```python
from build123d import *

# Parameters (mm, degrees)
SKETCH1_W           = 82
SKETCH1_H           = 37.5
BOSS_EXTRUDE2_DEPTH = 2
SKETCH2_W           = 3
SKETCH2_H           = 37.5
BOSS_EXTRUDE4_DEPTH = 3
BOSS_EXTRUDE5_DEPTH = 31
SKETCH6_W           = 16.5
SKETCH6_H           = 8
CUT_EXTRUDE1_DEPTH  = 2
SKETCH7_W           = 28.5
SKETCH7_H           = 25
CUT_EXTRUDE2_DEPTH  = 2
SKETCH8_W           = 0.8
SKETCH8_H           = 0.8
BOSS_EXTRUDE6_DEPTH = 5
SKETCH9_W           = 35
SKETCH9_H           = 2
BOSS_EXTRUDE7_DEPTH = 2.4


with BuildPart() as part:
    # Sketch1 → Boss-Extrude2 (new body)
    with BuildSketch(Plane(origin=(0, 0, 0), x_dir=(1, 0, 0), z_dir=(0, 1, 0))):
        with Locations((41, 18.75)):
            Rectangle(SKETCH1_W, SKETCH1_H)
    extrude(amount=BOSS_EXTRUDE2_DEPTH)

    # Sketch2 → Boss-Extrude4 (add)
    with BuildSketch(Plane(origin=(0, 2, 0), x_dir=(1, 0, 0), z_dir=(0, 1, 0))):
        with Locations((9.5, 18.75)):
            Rectangle(SKETCH2_W, SKETCH2_H)
        with Locations((68.5, 18.75)):
            Rectangle(SKETCH2_W, SKETCH2_H)
    extrude(amount=BOSS_EXTRUDE4_DEPTH)

    # Sketch4 → Boss-Extrude5 (add)
    with BuildSketch(Plane(origin=(0, 2, 0), x_dir=(1, 0, 0), z_dir=(0, 1, 0))):
        Polygon((11, 37.5), (8, 37.5), (0, 37.5), (0, 0), (8, 0), (11, 0), (67, 0), (70, 0), (82, 0), (82, 37.5), (70, 37.5), (67, 37.5), align=None)
        Polygon((2, 2), (2, 35.5), (8, 35.5), (11, 35.5), (67, 35.5), (70, 35.5), (80, 35.5), (80, 2), (70, 2), (67, 2), (11, 2), (8, 2), align=None, mode=Mode.SUBTRACT)
    extrude(amount=BOSS_EXTRUDE5_DEPTH)

    # Sketch6 → Cut-Extrude1 (cut)
    with BuildSketch(Plane.ZY):
        with Locations((-18.75, 29)):
            Rectangle(SKETCH6_W, SKETCH6_H)
    extrude(amount=-CUT_EXTRUDE1_DEPTH, mode=Mode.SUBTRACT)

    # Sketch7 → Cut-Extrude2 (cut)
    with BuildSketch(Plane(origin=(82, 0, 0), x_dir=(0, 0, -1), z_dir=(1, 0, 0))):
        with Locations((18.75, 17.5)):
            Rectangle(SKETCH7_W, SKETCH7_H)
    extrude(amount=-CUT_EXTRUDE2_DEPTH, mode=Mode.SUBTRACT)

    # Sketch8 → Boss-Extrude6 (add)
    with BuildSketch(Plane(origin=(2, 0, 0), x_dir=(0, 0, -1), z_dir=(1, 0, 0))):
        with Locations((7.65, 28.2)):
            Rectangle(SKETCH8_W, SKETCH8_H)
        with Locations((29.85, 28.2)):
            Rectangle(SKETCH8_W, SKETCH8_H)
    extrude(amount=BOSS_EXTRUDE6_DEPTH)

    # Sketch9 → Boss-Extrude7 (add)
    with BuildSketch(Plane(origin=(0, 0, -37.5), x_dir=(-1, 0, 0), z_dir=(0, 0, -1))):
        with Locations((-55.5, 26)):
            Rectangle(SKETCH9_W, SKETCH9_H)
        with Locations((-55.5, 5)):
            Rectangle(SKETCH9_W, SKETCH9_H)
    extrude(amount=BOSS_EXTRUDE7_DEPTH)


solid = part.part
```
Input: part model. Units: mm. Frame: model coordinates. A direction names the side the tool comes from. Give positions to 0.01 mm unless a question says otherwise; leave off trailing zeros. Order: outer loops, then holes, each group sorted by start corner. A loop starts at its lowest first (then second) coordinate and runs counter-clockwise, first axis right, second up. Notation, with made-up numbers: (39, -36.5) - (43, -36.5) arc R18 cw to (43, -28.5) - close; hole circle Ø10 at (48, -37.75). An arc over 180 degrees is marked (long way). Use a Markdown table: item, result.
(1) Section query B-B (x = 40). Output: boundary loops of the cut face in (y, z), then the cut area to 3 significant figures.
Computed values:
| item | result |
|---|---|
| outline | (0, -37.5) - (4, -37.5) - (4, -39.9) - (6, -39.9) - (6, -37.5) - (25, -37.5) - (25, -39.9) - (27, -39.9) - (27, -37.5) - (33, -37.5) - (33, -35.5) - (2, -35.5) - (2, -2) - (33, -2) - (33, 0) - (0, 0) - close |
| area | 209 mm2 |
(2) Draft query along Y for faces 6 (the flat face through (81, 17, -4.5)), 7 (the flat face through (75, 2, -19)), 8 (the flat face through (40, 17, -35.5)). Return one class per face: released by +Y, released by -Y, zero draft, split by the parting line, or undercut.
Computed values:
| item | result |
|---|---|
| face 6 | undercut |
| face 7 | released by +Y |
| face 8 | zero draft |
(3) Section query C-C (y = 9.5). Output: boundary loops of the cut face in (x, z).
Computed values:
| item | result |
|---|---|
| outline | (0, -37.5) - (82, -37.5) - (82, -33) - (80, -33) - (80, -35.5) - (2, -35.5) - (2, -2) - (80, -2) - (80, -4.5) - (82, -4.5) - (82, 0) - (0, 0) - close |
(4) Line query: line 1 (X direction, y = 30, z = -3.5); line 2 (Z direction, x = 33.5, y = 7.5); line 3 (Y direction, x = 29.5, z = -15.5). Output: solid intervals per line, ascending. Write a range as from..to.
Computed values:
| item | result |
|---|---|
| line 1 | x = 0..2, 80..82 |
| line 2 | z = -37.5..-35.5, -2..0 |
| line 3 | y = 0..2 |
(5) Section query D-D (x = 21). Output: boundary loops of the cut face in (y, z), then the cut area to 3 significant figures.
Computed values:
| item | result |
|---|---|
| outline | (0, -37.5) - (33, -37.5) - (33, -35.5) - (2, -35.5) - (2, -2) - (33, -2) - (33, 0) - (0, 0) - close |
| area | 199 mm2 |
(6) Access query for faces 1 (the flat face through (8, 3, -19)), 2 (the flat face through (56, 25, -39)), 3 (the flat face through (81, 5, -19)), 4 (the flat face through (1, 25, -19)), 5 (the flat face through (38, 5, -39)). Directions: +Z, -Z, +X, -X, +Y, -Y. A direction counts if a zero-diameter tool reaches every point of the face in a straight line with its end or side. Return the directions, or none.
Computed values:
| item | result |
|---|---|
| face 1 | +Y |
| face 2 | -Z, +X, -X |
| face 3 | +X |
| face 4 | +X, -X, +Y |
| face 5 | -Z, -X, +Y, -Y |
(7) Pin query (flat end, axial travel): pin 1 (2.5 mm diameter, centred on y = 3.5, z = -23.5, fed in from -X); pin 2 (0.6 mm diameter, centred on y = 26, z = -39, fed in from -X); pin 3 (1 mm diameter, centred on x = 1.5, z = -21.5, fed in from +Y); pin 4 (1.2 mm diameter, centred on x = 54.5, z = -39, fed in from -Y). Return the tip coordinate at first contact, or that it passes through.
Computed values:
| item | result |
|---|---|
| pin 1 | stops at x = 0 |
| pin 2 | stops at x = 38 |
| pin 3 | stops at y = 25 |
| pin 4 | stops at y = 4 |
(8) Section query A-A (z = -9.5). Output: boundary loops of the cut face in (x, y).
Computed values:
| item | result |
|---|---|
| outline | (0, 0) - (82, 0) - (82, 5) - (80, 5) - (80, 2) - (70, 2) - (70, 5) - (67, 5) - (67, 2) - (11, 2) - (11, 5) - (8, 5) - (8, 2) - (2, 2) - (2, 33) - (0, 33) - close; (80, 30) - (82, 30) - (82, 33) - (80, 33) - close |
